```python
from build123d import *

# Parameters (mm, degrees)
BOSS_EXTRUDE1_DEPTH         = 12.7
F_1_4_CLEARANCE_HOLE1_D     = 6.7564
F_1_4_CLEARANCE_HOLE1_DEPTH = 219.964
F_1_4_CLEARANCE_HOLE1_TIP   = 2.029827343
FILLET1_R                   = 12.7
FILLET2_R                   = 6.35


with BuildPart() as part:
    # Sketch1 → Boss-Extrude1 (new body)
    with BuildSketch(Plane.XY):
        Polygon((-114.3, -31.75), (-76.2, -31.75), (-76.2, 241.3), (76.2, 241.3), (76.2, -31.75), (114.3, -31.75), (114.3, 298.45), (76.2, 298.45), (76.2, 279.4), (-76.2, 279.4), (-76.2, 298.45), (-114.3, 298.45), align=None)
    extrude(amount=BOSS_EXTRUDE1_DEPTH)

    # 1/4 Clearance Hole1
    with Locations(Plane.XY.offset(12.7)):
        with Locations((-95.25, -11.1125), (-95.25, 9.525), (95.25, -11.1125), (95.25, 9.525)):
            Hole(F_1_4_CLEARANCE_HOLE1_D / 2, depth=F_1_4_CLEARANCE_HOLE1_DEPTH)
            with Locations((0, 0, -(F_1_4_CLEARANCE_HOLE1_DEPTH + F_1_4_CLEARANCE_HOLE1_TIP / 2))):  # 118° drill point
                Cone(0, F_1_4_CLEARANCE_HOLE1_D / 2, F_1_4_CLEARANCE_HOLE1_TIP, mode=Mode.SUBTRACT)

    # Fillet1
    fillet1_edges = [part.edges().sort_by_distance(p)[0] for p in [
        (-76.2, 279.4, 6.35),
        (76.2, 279.4, 6.35),
        (76.2, 241.3, 6.35),
        (-76.2, 241.3, 6.35),
    ]]
    fillet(fillet1_edges, radius=FILLET1_R)

    # Fillet2
    fillet2_edges = [part.edges().sort_by_distance(p)[0] for p in [
        (114.3, 298.45, 6.35),
        (76.2, 298.45, 6.35),
        (-114.3, 298.45, 6.35),
        (-76.2, 298.45, 6.35),
    ]]
    fillet(fillet2_edges, radius=FILLET2_R - 0.0001)  # a hair under: the kernel refuses the full size


solid = part.part
```
CAD build for the part. Positions are in the model's coordinates, mm. A direction names the side the tool comes from. Round coordinates to 2 decimals unless told otherwise and drop trailing zeros. Loops run counter-clockwise (first coordinate to the right, second up) from the corner with the lowest first, then second, coordinate; pieces in that order, holes last. Notation, with made-up numbers: M 86,-3.5 L 124,-3.5 A27 ccw 124,16.5 Z; hole C 47.25,12.5 d8. An arc over 180 degrees is marked long. Use a Markdown table: item, result. Add a question column.
(1) Which spindle directions (+Z, -Z, +X, -X, +Y, -Y) get a long thin tool onto all of the face, cutting with end or side? Do faces 4 (the face through (76.2, 100, 6)), 5 (the face through (92.028, 10.54, 6.261)), 6 (the face through (78.11, 296.64, 6.44)). Say none if no direction does.
(2) Drill centre lines: line 1 (Y direction, x = -95.25, z = 6); line 2 (X direction, y = 204, z = 10); line 3 (X direction, y = -14, z = 3). Where is each one in solid material? Low to high.
(3) Flat gauge pins, fed straight in: pin 1 (1.5 mm diameter, centred on x = -68.5, z = 6, fed in from +Y); pin 2 (1.5 mm diameter, centred on x = 10, z = 1.5, fed in from -Y). Where does each tip first touch, or does it go through?
(4) Cut at C-C (z = 8.25). State how many separate pieces and enclosed holes the cut face has, and give its area (3 significant figures).
(5) Cut at D-D (x = 46). Give the cut face in (y, z).
(6) Cut at A-A (y = 21.5). Give the cut face in (x, z), and give its area (3 significant figures).
(7) Cut at B-B (x = -95.25). Give the cut face in (y, z).
(8) Pull direction Y, two halves, no side cores. Call faces 1 (the face through (-96, -31.75, 6)), 2 (the face through (92.13, -12.41, 6.26)), 3 (the face through (112.49, 296.54, 6.44)): +Y half, -Y half, draft (parallel to the pull), parting line (faces both ways), or undercut.
Geometry says:
| question | item | result |
|---|---|---|
| 1 | face 4 | +Z, -Z, -Y |
| 1 | face 5 | +Z, -Z |
| 1 | face 6 | +Z, -Z, +Y |
| 2 | line 1 | y = -31.75 to -14.49, -7.73 to 6.15, 12.9 to 298.45 |
| 2 | line 2 | x = -114.3 to -76.2, 76.2 to 114.3 |
| 2 | line 3 | x = -114.3 to -97, -93.5 to -76.2, 76.2 to 93.5, 97 to 114.3 |
| 3 | pin 1 | stops at y = 280.78 |
| 3 | pin 2 | stops at y = 241.3 |
| 4 | separate pieces | 1 |
| 4 | enclosed holes | 4 |
| 4 | area | 30,900 mm² |
| 5 | outline | M 241.3,0 L 279.4,0 L 279.4,12.7 L 241.3,12.7 Z |
| 6 | outline | M -114.3,0 L -76.2,0 L -76.2,12.7 L -114.3,12.7 Z; M 76.2,0 L 114.3,0 L 114.3,12.7 L 76.2,12.7 Z |
| 6 | area | 968 mm² |
| 7 | outline | M -31.75,0 L -14.49,0 L -14.49,12.7 L -31.75,12.7 Z; M -7.73,0 L 6.15,0 L 6.15,12.7 L -7.73,12.7 Z; M 12.9,0 L 298.45,0 L 298.45,12.7 L 12.9,12.7 Z |
| 8 | face 1 | -Y half |
| 8 | face 2 | undercut |
| 8 | face 3 | +Y half |
